Autodesk Inventor part; units mm, degrees
ref_plane "h1_XY" through (-102.3874, 0, 0) normal (0, 1, 0) x (1, 0, 0)
ref_plane "h1_YZ" through (-102.3874, 0, 0) normal (1, 0, 0) x (0, 0, -1)
ref_plane "h1_ZX" through (-102.3874, 0, 0) normal (0, 0, -1) x (0, 1, 0)
sketch "Sketch_3" plane through (0, 0, 0) normal (0, 0, 1) x (1, 0, 0)
  line L0 (0, 0) -> (-102.3874, 0)
  line L1 (-102.3874, 0) -> (-102.3874, 1.9406)
  line L2 (-102.3874, 1.9406) -> (-101.915, 2.413)
  line L3 (-101.915, 2.413) -> (0, 2.413)
  line L4 (0, 2.413) -> (0, 0)
  line L5 (0, 0) -> (-102.3874, 0)
revolve "Revolution1" add sketch "Sketch_3" angle 360 about axis through (0, 0, 0) along (1, 0, 0)
thread "Thread1"
sketch "Sketch_17" plane through (0, 0, 0) normal (0, 0, 1) x (1, 0, 0)
  line L0 (102.3874, 0) -> (-102.3874, 0)
  line L1 (-89.9414, 2.413) -> (-89.9414, 2.159)
  line L2 (-89.9414, 2.159) -> (-89.6874, 2.159)
  line L3 (-89.6874, 2.159) -> (-89.6874, 2.413)
  line L4 (-89.6874, 2.413) -> (-89.9414, 2.413)
revolve "Revolution2" cut sketch "Sketch_17" angle 360 about axis through (102.3874, 0, 0) along (1, 0, 0)
sketch "Sketch_12" plane through (0, 0, 0) normal (0, 0, 1) x (1, 0, 0)
  line L0 (1.524, 0) -> (-15.875, 0)
  line L1 (-15.875, 0) -> (-15.875, 7.2771)
  line L2 (-15.875, 7.2771) -> (1.524, 7.2771)
  line L3 (1.524, 7.2771) -> (1.524, 0)
  line L4 (1.524, 0) -> (-15.875, 0)
revolve "Revolution3" add sketch "Sketch_12" angle 360 about axis through (1.524, 0, 0) along (1, 0, 0)
ref_plane "h1_XY" through (-102.3874, 0, 0) normal (0, 1, 0) x (1, 0, 0)
ref_plane "h1_YZ" through (-102.3874, 0, 0) normal (1, 0, 0) x (0, 0, -1)
ref_plane "h1_ZX" through (-102.3874, 0, 0) normal (0, 0, -1) x (0, 1, 0)
ref_plane "h2_XY" through (-89.6874, 0, 0) normal (0, 1, 0) x (1, 0, 0)
ref_plane "h2_YZ" through (-89.6874, 0, 0) normal (1, 0, 0) x (0, 0, -1)
ref_plane "h2_ZX" through (-89.6874, 0, 0) normal (0, 0, -1) x (0, 1, 0)
ref_plane "k1_XY" through (-102.3874, 0, -2.413) normal (0, 1, 0) x (1, 0, 0)
ref_plane "k1_YZ" through (-102.3874, 0, -2.413) normal (1, 0, 0) x (0, 0, -1)
ref_plane "k1_ZX" through (-102.3874, 0, -2.413) normal (0, 0, -1) x (0, 1, 0)
ref_plane "k2_XY" through (-102.3874, 0, 2.413) normal (0, 1, 0) x (1, 0, 0)
ref_plane "k2_YZ" through (-102.3874, 0, 2.413) normal (1, 0, 0) x (0, 0, -1)
ref_plane "k2_ZX" through (-102.3874, 0, 2.413) normal (0, 0, -1) x (0, 1, 0)
ref_plane "start_XY" through (-89.6874, 0, 0) normal (0, 1, 0) x (1, 0, 0)
ref_plane "start_YZ" through (-89.6874, 0, 0) normal (1, 0, 0) x (0, 0, -1)
ref_plane "start_ZX" through (-89.6874, 0, 0) normal (0, 0, -1) x (0, 1, 0)
ref_plane "to_prc_XY" through (-89.6874, 0, 0) normal (1, 0, 0) x (0, 0, -1)
ref_plane "to_prc_YZ" through (-89.6874, 0, 0) normal (0, 0, -1) x (0, 1, 0)
ref_plane "to_prc_ZX" through (-89.6874, 0, 0) normal (0, 1, 0) x (1, 0, 0)
ref_plane "to_rod_guide_XY" through (-102.3874, 0, 0) normal (1, 0, 0) x (0, 0, -1)
ref_plane "to_rod_guide_YZ" through (-102.3874, 0, 0) normal (0, 0, -1) x (0, 1, 0)
ref_plane "to_rod_guide_ZX" through (-102.3874, 0, 0) normal (0, 1, 0) x (1, 0, 0)
properties part number "D-75081.5-0.25-4.031-3pos"
The listing builds one solid part. Answer for the finished solid, in the listing's coordinates (mm). A direction names the side the tool comes from. Give positions to 0.01 mm unless a question says otherwise; leave off trailing zeros. Order: outer loops, then holes, each group sorted by start corner. A loop starts at its lowest first (then second) coordinate and runs counter-clockwise, first axis right, second up.
Item 1: The part is cut by section D-D, the plane y = -3.75. Give the vertices of the cut face in (x, z) (3 decimals), and give its area (3 significant figures).
From the geometry:
outline: (-15.875, -6.236) - (1.524, -6.236) - (1.524, 6.236) - (-15.875, 6.236) - close
area: 217 mm2
Item 2: Find the intervals of material crossed by probe 1 along X at (y, z) = (-5.75, 3.5) (3 decimals); probe 2 along Y at (x, z) = (-63.5, -0.25); probe 3 along Z at (x, y) = (-25, 1.75), in increasing order.
From the geometry:
probe 1: x = -15.875 to 1.524
probe 2: y = -2.4 to 2.4
probe 3: z = -1.66 to 1.66
Item 3: Which of the six approach directions +Z, -Z, +X, -X, +Y, -Y give full straight-line access (tool end or side, diameter ignored) to faces 1 (the face through (-95.844, -1.915, -1.468)), 2 (the face through (1.524, 0, 0))?
From the geometry:
face 1: -X
face 2: +Z, -Z, +X, +Y, -Y
Item 4: Given pin 1 Ø1.5 at (x, y) = (-75, 2.5) entering from -Z; pin 2 Ø2 at (x, z) = (-39.5, 3.5) entering from +Y; pin 3 Ø4 at (x, z) = (-9.5, 0.5) entering from +Y; pin 4 Ø6 at (x, y) = (-83.5, 4.5) entering from +Z, each flat-ended and moving along its own axis, determine where each tip first touches the part or whether it passes through.
From the geometry:
pin 1: stops at z = -1.66
pin 2: passes through
pin 3: stops at y = 7.28
pin 4: stops at z = 1.89
Item 5: The part is cut by section A-A, the plane y = 0. Give the vertices of the cut face in (x, z) (3 decimals), and give its area (3 significant figures).
From the geometry:
outline: (-102.387, -1.941) - (-101.915, -2.413) - (-89.941, -2.413) - (-89.941, -2.159) - (-89.687, -2.159) - (-89.687, -2.413) - (-15.875, -2.413) - (-15.875, -7.277) - (1.524, -7.277) - (1.524, 7.277) - (-15.875, 7.277) - (-15.875, 2.413) - (-89.687, 2.413) - (-89.687, 2.159) - (-89.941, 2.159) - (-89.941, 2.413) - (-101.915, 2.413) - (-102.387, 1.941) - close
area: 670 mm2
Item 6: The part is cut by section C-C, the plane x = -61. Give the vertices of the cut face in (y, z), and give its area (3 significant figures).
From the geometry:
outline: circle Ø4.83 at (0, 0)
area: 18.3 mm2
